```python
from build123d import *

# Parameters (mm, degrees)
F0_W     = 62.650863
F0_H     = 45.193966
F1_DEPTH = 25
F2_R     = 10.595561
F3_DEPTH = 25
F4_R     = 6.563376
F5_DEPTH = 25


with BuildPart() as f1:
    # F0 (on Front) → F1 (new body)
    with BuildSketch(Plane.XZ):
        with Locations((9.019395, -0.67888)):
            Rectangle(F0_W, F0_H)
    extrude(amount=F1_DEPTH)

    # F2 (on face) → F3 (cut)
    with BuildSketch(Plane.XZ.offset(25)):
        with Locations((1.551725, 0)):
            Circle(F2_R)
    extrude(amount=-F3_DEPTH, mode=Mode.SUBTRACT)

    # F4 (on face) → F5 (join)
    with BuildSketch(Plane.XZ.offset(25)):
        with Locations((26.767241, 0)):
            Circle(F4_R)
    extrude(amount=-F5_DEPTH)


solid = f1.part
```
Build history of the part. All positions in model axes, mm. Coordinates: 2 decimals unless noted, no trailing zeros. Order: outer loops, then holes, each group sorted by start corner. A loop starts at its lowest first (then second) coordinate and runs counter-clockwise, first axis right, second up. Notation, with made-up numbers: (88.5, -12.5) -> (111.5, -12.5) arc R28 cw to (111.5, 6.5) -> close; hole circle Ø8 at (11.25, -5). An arc over 180 degrees is marked (long way). Answer in a Markdown table with one row per item. Add a question column.
Q1. Wall check: line 1 along Z through (x, y) = (4, -17.25); line 2 along Z through (x, y) = (2.5, -6.25); line 3 along X through (y, z) = (-22.5, -6). Give the ranges that are in metal, low to high. Write a range as [from, to].
Q2. Band-saw the part on A-A, the plane z = 0. List the corners of the cut face in (x, y), then the cut area to 3 significant figures.
Q3. Band-saw the part on B-B, the plane y = -5. List the corners of the cut face in (x, z), then the cut area to 3 significant figures.
Q4. Band-saw the part on C-C, the plane x = 8. List the corners of the cut face in (y, z), then the cut area to 3 significant figures.
Answers follow:
| question | item | result |
|---|---|---|
| 1 | line 1 | [-23.28, -10.31], [10.31, 21.92] |
| 1 | line 2 | [-23.28, -10.55], [10.55, 21.92] |
| 1 | line 3 | [-22.31, -7.18], [10.28, 40.34] |
| 2 | outline | (-22.31, -25) -> (-9.04, -25) -> (-9.04, 0) -> (-22.31, 0) -> close; (12.15, -25) -> (40.34, -25) -> (40.34, 0) -> (12.15, 0) -> close |
| 2 | area | 1,040 mm^2 |
| 3 | outline | (-22.31, -23.28) -> (40.34, -23.28) -> (40.34, 21.92) -> (-22.31, 21.92) -> close; hole circle Ø21.19 at (1.55, 0) |
| 3 | area | 2,480 mm^2 |
| 4 | outline | (-25, -23.28) -> (0, -23.28) -> (0, -8.41) -> (-25, -8.41) -> close; (-25, 8.41) -> (0, 8.41) -> (0, 21.92) -> (-25, 21.92) -> close |
| 4 | area | 709 mm^2 |
